The model under review builds one solid part; all positions refer to its coordinate system, in mm. Face numbers are marked on the shaded views. Round coordinates to 2 decimals unless told otherwise and drop trailing zeros. Loops run counter-clockwise (first coordinate to the right, second up) from the corner with the lowest first, then second, coordinate; pieces in that order, holes last. Notation, with made-up numbers: (49.25, -18.75) -> (53.25, -18.75) arc R28 ccw to (53.25, 3.25) -> close; hole circle Ø2 at (79, 64). An arc over 180 degrees is marked (long way). Use CSV: the item, a comma, the result in double quotes. Start each with the question number.
```python
from build123d import *

# Parameters (mm, degrees)
SKETCH1_W           = 43
SKETCH1_H           = 57
BOSS_EXTRUDE1_DEPTH = 4
SKETCH2_R           = 4
CUT_EXTRUDE1_DEPTH  = 37.58551626
FILLET1_R           = 3


with BuildPart() as part:
    # Sketch1 → Boss-Extrude1 (new, symmetric)
    with BuildSketch(Plane.XY):
        Rectangle(SKETCH1_W, SKETCH1_H)
    extrude(amount=BOSS_EXTRUDE1_DEPTH, both=True)

    # Sketch2 → Cut-Extrude1 (cut, through all)
    with BuildSketch(Plane.XY.offset(4)):
        with Locations((0, 13.5)):
            Circle(SKETCH2_R)
    extrude(amount=-CUT_EXTRUDE1_DEPTH, mode=Mode.SUBTRACT)

    # Fillet1
    fillet1_edges = [part.edges().sort_by_distance(p)[0] for p in [
        (21.5, -28.5, 0),
        (-21.5, -28.5, 0),
        (-21.5, 28.5, 0),
        (21.5, 28.5, 0),
    ]]
    fillet(fillet1_edges, radius=FILLET1_R)


solid = part.part
```
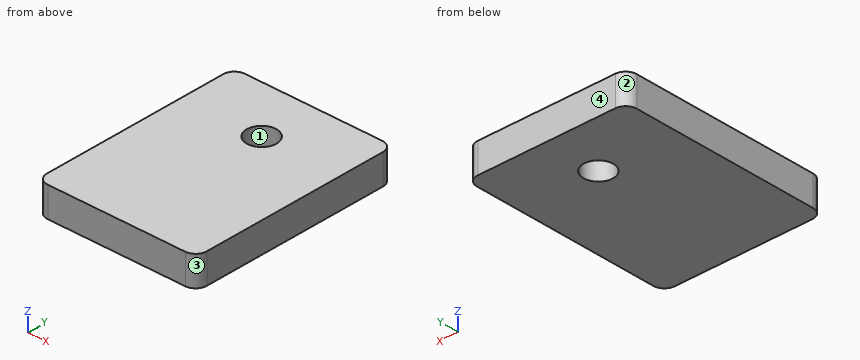
1. Take a section at A-A, the plane x = 0. Give the boundary of the cut face in (y, z).
2. The part is to be moulded in two halves that separate along X. For the marked faces 1, 2, 3 and 4, say which applies: pulls with the +X half, pulls with the -X half, needs draft (parallel to the pull), parting line crosses it, or undercut.
3. Take a section at C-C, the plane y = 13.5. Give the boundary of the cut face in (x, z), then the cut area to 3 significant figures.
4. For line 1 along Y through (x, z) = (0, -0.5), list the stretches that pass through material, from the lowest coordinate up. Write a range as from..to.
5. Take a section at B-B, the plane z = -0.5. Give the boundary of the cut face in (x, y).
Results:
1,outline,"(-28.5, -4) -> (9.5, -4) -> (9.5, 4) -> (-28.5, 4) -> close; (17.5, -4) -> (28.5, -4) -> (28.5, 4) -> (17.5, 4) -> close"
2,face 1,"undercut"
2,face 2,"pulls with the -X half"
2,face 3,"pulls with the +X half"
2,face 4,"needs draft"
3,outline,"(-21.5, -4) -> (-4, -4) -> (-4, 4) -> (-21.5, 4) -> close; (4, -4) -> (21.5, -4) -> (21.5, 4) -> (4, 4) -> close"
3,area,"280 mm²"
4,line 1,"-28.5..9.5, 17.5..28.5"
5,outline,"(-21.5, -25.5) arc R3 ccw to (-18.5, -28.5) -> (18.5, -28.5) arc R3 ccw to (21.5, -25.5) -> (21.5, 25.5) arc R3 ccw to (18.5, 28.5) -> (-18.5, 28.5) arc R3 ccw to (-21.5, 25.5) -> close; hole circle Ø8 at (0, 13.5)"
